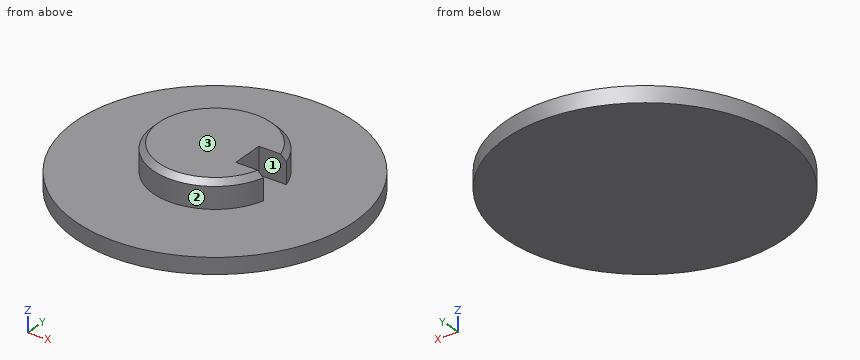
```python
from build123d import *

# Parameters (mm, degrees)
BOX211_W                         = 6
BOX211_H                         = 6
BOX211_DEPTH                     = 5
CYLINDER014005814004018007_R     = 26
CYLINDER014005814004018007_DEPTH = 3
CYLINDER014005814004018006_R     = 11.5
CYLINDER014005814004018006_DEPTH = 7
CHAMFER_SIZE                     = 1


with BuildPart() as krychle186:
    # Box211 → Box211 (new body)
    with BuildSketch(Plane(origin=(6, -3, 2), x_dir=(1, 0, 0), z_dir=(0, 0, 1))):
        with Locations((3, 3)):
            Rectangle(BOX211_W, BOX211_H)
    extrude(amount=BOX211_DEPTH)


with BuildPart() as obj1:
    # Cylinder014005814004018007 → Cylinder014005814004018007 (new body)
    with BuildSketch(Plane.XY.offset(-1)):
        Circle(CYLINDER014005814004018007_R)
    extrude(amount=CYLINDER014005814004018007_DEPTH)


with BuildPart() as cap2:
    # Cylinder014005814004018006 → Cylinder014005814004018006 (new body)
    with BuildSketch(Plane.XY):
        Circle(CYLINDER014005814004018006_R)
    extrude(amount=CYLINDER014005814004018006_DEPTH)

    # Fusion001089091: union obj1
    add(obj1.part)

    # Cut061098126006: cut Krychle186
    add(krychle186.part, mode=Mode.SUBTRACT)

    # Chamfer
    chamfer_edges = [cap2.edges().sort_by_distance(p)[0] for p in [
        (-11.5, 0, 7),
    ]]
    chamfer(chamfer_edges, length=CHAMFER_SIZE)


solid = cap2.part
```
CAD build for the part. Positions are in the model's coordinates, mm. Face numbers are marked on the shaded views. Coordinates: 2 decimals unless noted, no trailing zeros. Order: outer loops, then holes, each group sorted by start corner. A loop starts at its lowest first (then second) coordinate and runs counter-clockwise, first axis right, second up. Notation, with made-up numbers: (24.25, 54) - (30.25, 54) arc R16 cw to (30.25, 73) - close; hole circle Ø6 at (-37, 40). An arc over 180 degrees is marked (long way). Answer in a Markdown table with one row per item.
1. Flat gauge pins, fed straight in: P1, Ø15.5, axis at x = -9.5, y = 12, coming from the +Z side; P2, Ø4, axis at x = 9.5, z = 5, coming from the +Y side; P3, Ø2.5, axis at x = 8.5, z = 4, coming from the -Y side; P4, Ø2, axis at y = -9, z = 0.5, coming from the +X side. Where does each tip first touch, or does it go through?
Answer:
| item | result |
|---|---|
| P1 | z = 7 |
| P2 | y = 8.72 |
| P3 | y = -8.93 |
| P4 | x = 24.74 |
2. Drill centre lines: L1, parallel to Z at x = -8.5, y = -16; L2, parallel to X at y = -15, z = 1; L3, parallel to X at y = -7.5, z = 3.25. Where is each one in solid material? Low to high. Write a range as from..to.
Answer:
| item | result |
|---|---|
| L1 | -1..2 |
| L2 | -21.24..21.24 |
| L3 | -8.72..8.72 |
3. Slice it at A-A, the plane x = 0. List the corners of the cut face in (y, z).
Answer:
| item | result |
|---|---|
| outline | (-26, -1) - (26, -1) - (26, 2) - (11.5, 2) - (11.5, 6) - (10.5, 7) - (-10.5, 7) - (-11.5, 6) - (-11.5, 2) - (-26, 2) - close |
4. Pull direction Y, two halves, no side cores. Call the marked faces 1, 2 and 3: +Y half, -Y half, draft (parallel to the pull), parting line (faces both ways), or undercut.
Answer:
| item | result |
|---|---|
| face 1 | undercut |
| face 2 | parting line |
| face 3 | draft |
5. Slice it at C-C, the plane z = 4.5. List the corners of the cut face in (x, y).
Answer:
| item | result |
|---|---|
| outline | (6, -3) - (6, 3) - (11.1, 3) arc R11.5 ccw (long way) to (11.1, -3) - close |
6. Slice it at D-D, the plane y = -17.5. List the corners of the cut face in (x, z), then the cut area to 3 significant figures.
Answer:
| item | result |
|---|---|
| outline | (-19.23, -1) - (19.23, -1) - (19.23, 2) - (-19.23, 2) - close |
| area | 115 mm² |
7. Slice it at B-B, the plane y = 0. List the corners of the cut face in (x, z).
Answer:
| item | result |
|---|---|
| outline | (-26, -1) - (26, -1) - (26, 2) - (6, 2) - (6, 7) - (-10.5, 7) - (-11.5, 6) - (-11.5, 2) - (-26, 2) - close |
